```python
from build123d import *

# Parameters (mm, degrees)
F1_DEPTH       = 19.05
F3_D           = 9.525
F3_CBORE_D     = 15.875
F3_CBORE_DEPTH = 9.525


# Not quite as in the source:
# - a length typed as a fraction of an inch, garbled in the dataset ("3 / 203.2 mm" for 3/8 in), is restored


with BuildPart() as f1:
    # F0 (on Front) → F1 (new body, symmetric)
    with BuildSketch(Plane.XZ):
        Polygon((-50.8, 0), (0, 0), (0, 50.8), (-22.225, 50.8), (-22.225, 31.75), (-69.85, 31.75), (-69.85, 19.05), (-50.8, 19.05), align=None)
    extrude(amount=F1_DEPTH, both=True)

    # F3 (through all)
    with Locations(Plane.YZ):
        with Locations((-9.525, 9.525), (9.525, 9.525)):
            CounterBoreHole(F3_D / 2, F3_CBORE_D / 2, F3_CBORE_DEPTH)


solid = f1.part
```
Design review of the part built by this model. Coordinates are the model's own, in mm. A direction names the side the tool comes from. Give positions to 0.01 mm unless a question says otherwise; leave off trailing zeros. Loops run counter-clockwise (first coordinate to the right, second up) from the corner with the lowest first, then second, coordinate; pieces in that order, holes last. Notation, with made-up numbers: (49, -31) -> (53, -31) arc R13 ccw to (53, -6) -> close; hole circle Ø2 at (-15.5, -35.75). An arc over 180 degrees is marked (long way). One line per item, written item: value.
Q1. Draft analysis for pull direction Z (two halves, no side actions). For faces 4 (the flat face through (-26, 0, 0)), 5 (the flat face through (-22.225, 0, 41)), 6 (the flat face through (-9.525, -6, 6)), state which applies: pulls with the +Z half, pulls with the -Z half, needs draft (parallel to the pull), parting line crosses it, or undercut.
Numbers:
face 4: pulls with the -Z half
face 5: needs draft
face 6: undercut
Q2. We need section A-A on y = -10. Give the boundary of the cut face in (x, z) (3 decimals), and give its area (3 significant figures).
Numbers:
outline: (-69.85, 19.05) -> (-50.8, 19.05) -> (-50.8, 14.264) -> (-9.525, 14.264) -> (-9.525, 17.448) -> (0, 17.448) -> (0, 50.8) -> (-22.225, 50.8) -> (-22.225, 31.75) -> (-69.85, 31.75) -> close; (-50.8, 0) -> (0, 0) -> (0, 1.602) -> (-9.525, 1.602) -> (-9.525, 4.786) -> (-50.8, 4.786) -> close
area: 1,740 mm^2
Q3. For L1, parallel to Y at x = -40, z = 13.5; L2, parallel to X at y = 10, z = 36 (3 decimals); L3, parallel to Y at x = -11, z = 10, list the stretches that pass through material, from the lowest coordinate up.
Numbers:
L1: y = -19.05 to -12.15, -6.9 to 6.9, 12.15 to 19.05
L2: x = -22.225 to 0
L3: y = -19.05 to -14.26, -4.79 to 4.79, 14.26 to 19.05
Q4. For pin 1 Ø12.5 at (y, z) = (9.525, 9.525) entering from -X; pin 2 Ø2 at (x, y) = (-17, -3) entering from -Z; pin 3 Ø5 at (y, z) = (6.5, 6) entering from +X (3 decimals); pin 4 Ø5.5 at (x, y) = (-56, 5) entering from -Z, all flat-tipped, find the tip position at first contact; note any pin that passes through.
Numbers:
pin 1: stops at x = -50.8
pin 2: stops at z = 0
pin 3: stops at x = -9.525
pin 4: stops at z = 19.05
Q5. We need section D-D on z = 16.5. Give the boundary of the cut face in (x, y) (3 decimals).
Numbers:
outline: (-50.8, -19.05) -> (0, -19.05) -> (0, -13.314) -> (-9.525, -13.314) -> (-9.525, -5.736) -> (0, -5.736) -> (0, 5.736) -> (-9.525, 5.736) -> (-9.525, 13.314) -> (0, 13.314) -> (0, 19.05) -> (-50.8, 19.05) -> close
Q6. We need section B-B on y = 0.5. Give the boundary of the cut face in (x, z) (3 decimals).
Numbers:
outline: (-69.85, 19.05) -> (-50.8, 19.05) -> (-50.8, 0) -> (0, 0) -> (0, 50.8) -> (-22.225, 50.8) -> (-22.225, 31.75) -> (-69.85, 31.75) -> close
Q7. Machinability: for faces 1 (the flat face through (-9.525, 13, 6)), 2 (the flat face through (-46, 0, 31.75)), 3 (the flat face through (-50.8, 0, 10)), which of the approach directions +Z, -Z, +X, -X, +Y, -Y give a long, thin tool a straight path to every point of the face, cutting with its end or side? Answer none if there is none.
Numbers:
face 1: +X
face 2: +Z, -X, +Y, -Y
face 3: -Z, -X, +Y, -Y
Q8. We need section C-C on x = -39.5. Give the number of separate pieces and of enclosed holes in the cut face, and give its area (3 significant figures).
Numbers:
separate pieces: 1
enclosed holes: 2
area: 1,070 mm^2
